Model file for the job. Use its own axes, mm. A direction names the side the tool comes from. Round coordinates to 2 decimals unless told otherwise and drop trailing zeros. Order: outer loops, then holes, each group sorted by start corner. A loop starts at its lowest first (then second) coordinate and runs counter-clockwise, first axis right, second up. Notation, with made-up numbers: (71.25, 13) - (102.25, 13) arc R25 cw to (102.25, 45) - close; hole circle Ø8 at (70.25, 86). An arc over 180 degrees is marked (long way). Write item = value, one per line. Start each with the question number.
from build123d import *

# Parameters (mm, degrees)
ESQUISSE1_R        = 4.5
ESQUISSE1_R_2      = 1.1
BOSS_EXTRU_1_DEPTH = 4
SKETCH1_R          = 2.1
CUT_EXTRUDE1_DEPTH = 43.574273021


with BuildPart() as part:
    # Esquisse1 → Boss.-Extru.1 (new body)
    with BuildSketch(Plane.XY):
        with BuildLine():
            Line((-15, 3), (-15, 7))
            Line((-15, 7), (-5, 7))
            Line((-5, 7), (-5, 0))
            Line((-5, 0), (5, 0))
            Line((5, 0), (5, 7))
            Line((5, 7), (15, 7))
            Line((15, 7), (15, 3))
            Line((15, 3), (15, -13.574063778))
            Line((15, -13.574063778), (10.686419419, -31.250781398))
            ThreePointArc((10.686419419, -31.250781398), (0, -39.643016072), (-10.686419419, -31.250781398))
            Line((-10.686419419, -31.250781398), (-15, -13.574063778))
            Line((-15, -13.574063778), (-15, 3))
        make_face()
        with Locations((0, -28.643016072)):
            Circle(ESQUISSE1_R, mode=Mode.SUBTRACT)
        with Locations((0, -21.643016072)):
            Circle(ESQUISSE1_R_2, mode=Mode.SUBTRACT)
        with Locations((4.949747468, -23.693268604)):
            Circle(ESQUISSE1_R_2, mode=Mode.SUBTRACT)
        with Locations((7, -28.643016072)):
            Circle(ESQUISSE1_R_2, mode=Mode.SUBTRACT)
        with Locations((4.949747468, -33.59276354)):
            Circle(ESQUISSE1_R_2, mode=Mode.SUBTRACT)
        with Locations((0, -35.643016072)):
            Circle(ESQUISSE1_R_2, mode=Mode.SUBTRACT)
        with Locations((-4.949747468, -33.59276354)):
            Circle(ESQUISSE1_R_2, mode=Mode.SUBTRACT)
        with Locations((-7, -28.643016072)):
            Circle(ESQUISSE1_R_2, mode=Mode.SUBTRACT)
        with Locations((-4.949747468, -23.693268604)):
            Circle(ESQUISSE1_R_2, mode=Mode.SUBTRACT)
    extrude(amount=BOSS_EXTRU_1_DEPTH)

    # Sketch1 → Cut-Extrude1 (cut, through all)
    with BuildSketch(Plane(origin=(0, 0, 0), x_dir=(-1, 0, 0), z_dir=(0, 0, -1))):
        with Locations((-9.368015407, 3.5)):
            Circle(SKETCH1_R)
        with Locations((9.663609861, 3.5)):
            Circle(SKETCH1_R)
    extrude(amount=-CUT_EXTRUDE1_DEPTH, mode=Mode.SUBTRACT)


solid = part.part
Item 1: Probe L1, parallel to Y at x = 0, z = 0.95; L2, parallel to X at y = 4, z = 3.7; L3, parallel to X at y = -25, z = 0.45. List the from-to ranges inside material, lowest first.
Item 2: Drop flat-ended pins along their axis: pin 1 (2.5 mm diameter, centred on x = -4.95, y = -33.59, fed in from -Z); pin 2 (1 mm diameter, centred on y = -22, z = 2, fed in from -X); pin 3 (1.2 mm diameter, centred on x = -1, z = 2.5, fed in from +Y). Give the stop position or say it passes through.
Item 3: Saw through at B-B, the plane x = 0. Give the cut face in (y, z), then the cut area to 3 significant figures.
Item 4: Saw through at C-C, the plane x = -7. Give the cut face in (y, z).
Item 5: Saw through at A-A, the plane y = 3.5. Give the cut face in (x, z).
Item 6: Saw through at D-D, the plane z = 2.5. Give the number of separate pieces and of enclosed holes in the cut face, then the cut area to 3 significant figures.
Item 7: Which spindle directions (+Z, -Z, +X, -X, +Y, -Y) get a long thin tool onto all of the face, cutting with end or side? Do faces 1 (the face through (-12.813, -22.536, 1.972)), 2 (the face through (5, 3, 2)). Say none if no direction does.
Check sheet entries:
q1.L1 = -39.64 to -36.74, -34.54 to -33.14, -24.14 to -22.74, -20.54 to 0
q1.L2 = -15 to -11.7, -7.62 to -5, 5 to 7.33, 11.41 to 15
q1.L3 = -12.21 to -2.64, 2.64 to 12.21
q2.pin_1 = 0
q2.pin_2 = -13.07
q2.pin_3 = 0
q3.outline = (-39.64, 0) - (-36.74, 0) - (-36.74, 4) - (-39.64, 4) - close; (-34.54, 0) - (-33.14, 0) - (-33.14, 4) - (-34.54, 4) - close; (-24.14, 0) - (-22.74, 0) - (-22.74, 4) - (-24.14, 4) - close; (-20.54, 0) - (0, 0) - (0, 4) - (-20.54, 4) - close
q3.area = 105 mm2
q4.outline = (-37.13, 0) - (-29.74, 0) - (-29.74, 4) - (-37.13, 4) - close; (-27.54, 0) - (7, 0) - (7, 4) - (-27.54, 4) - close
q5.outline = (-15, 0) - (-11.76, 0) - (-11.76, 4) - (-15, 4) - close; (-7.56, 0) - (-5, 0) - (-5, 4) - (-7.56, 4) - close; (5, 0) - (7.27, 0) - (7.27, 4) - (5, 4) - close; (11.47, 0) - (15, 0) - (15, 4) - (11.47, 4) - close
q6.separate_pieces = 1
q6.enclosed_holes = 11
q6.area = 1,010 mm2
q7.face_1 = +Z, -Z, -X, -Y
q7.face_2 = +Z, -Z, +Y
